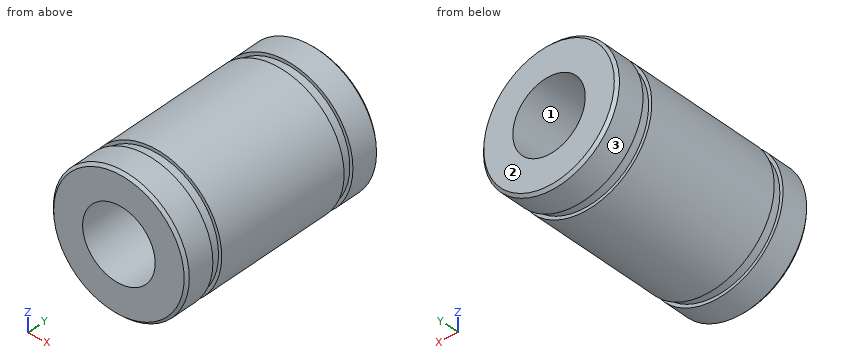
Autodesk Fusion 360 part; units mm, degrees
sketch "Sketch1" plane through (0, 0, 0) normal (0, 1, 0) x (1, 0, 0)
  circle A0 centre (0, 0) radius 4
  circle A1 centre (0, 0) radius 7.5
  circle A2 centre (0, 0) radius 7.15
  dimension "d1" = 8
  dimension "d2" = 15
  dimension "d6" = 0.35
extrude "Extrude1" add sketch "Sketch1" along normal blind 24 contours A1 | A2
extrude "Extrude2" cut sketch "Sketch1" along normal blind 1.1 from surface at 3.25 contours A1
extrude "Extrude3" cut sketch "Sketch1" against normal blind 1.1 from surface at 20.75 contours A1
chamfer "Chamfer1" distance 0.3 angle 45 2 edges at (-6.9925, 0, 2.7121) (-6.9925, 24, 2.7121)
Verification items for the finished model (mm, model axes). Face numbers are marked on the shaded views. Give positions to 0.01 mm unless a question says otherwise; leave off trailing zeros. Write each loop counter-clockwise with the first axis right and the second up, starting at its lowest first coordinate (ties: lowest second). Pieces come first, ordered by that corner, then holes. Notation, with made-up numbers: M -5.75,-13.5 L 9.25,-13.5 A21 ccw 9.25,23.5 Z; hole C 57.5,52 d3. An arc over 180 degrees is marked long. Write item = value, one per line.
(1) Sectioned sample at A-A (z = 0). Record the cut outline in (x, y), then the cut area to 3 significant figures.
Found:
outline = M -7.5,0.3 L -7.2,0 L -4,0 L -4,24 L -7.2,24 L -7.5,23.7 L -7.5,20.75 L -7.15,20.75 L -7.15,19.65 L -7.5,19.65 L -7.5,4.35 L -7.15,4.35 L -7.15,3.25 L -7.5,3.25 Z; M 4,0 L 7.2,0 L 7.5,0.3 L 7.5,3.25 L 7.15,3.25 L 7.15,4.35 L 7.5,4.35 L 7.5,19.65 L 7.15,19.65 L 7.15,20.75 L 7.5,20.75 L 7.5,23.7 L 7.2,24 L 4,24 Z
area = 166 mm2
(2) Sectioned sample at B-B (x = 0). Record the cut outline in (y, z), then the cut area to 3 significant figures.
Found:
outline = M 0,-7.2 L 0.3,-7.5 L 3.25,-7.5 L 3.25,-7.15 L 4.35,-7.15 L 4.35,-7.5 L 19.65,-7.5 L 19.65,-7.15 L 20.75,-7.15 L 20.75,-7.5 L 23.7,-7.5 L 24,-7.2 L 24,-4 L 0,-4 Z; M 0,4 L 24,4 L 24,7.2 L 23.7,7.5 L 20.75,7.5 L 20.75,7.15 L 19.65,7.15 L 19.65,7.5 L 4.35,7.5 L 4.35,7.15 L 3.25,7.15 L 3.25,7.5 L 0.3,7.5 L 0,7.2 Z
area = 166 mm2
(3) Material ranges on line 1 (X direction, y = 17, z = 0); line 2 (X direction, y = 13.75, z = 3.5), recorded low to high.
Found:
line_1 = -7.5 to -4, 4 to 7.5
line_2 = -6.63 to -1.94, 1.94 to 6.63
(4) Go/stop test with flat-tipped pins: pin 1 Ø5 at (x, y) = (3, 6) entering from -Z; pin 2 Ø1.5 at (x, z) = (-1, -3) entering from +Y; pin 3 Ø3 at (x, y) = (-3, 18) entering from +Z. Record where each tip stops, or that it passes through.
Found:
pin_1 = -7.48
pin_2 = through
pin_3 = 7.35
(5) Sectioned sample at C-C (y = 3.75). Record the cut outline in (x, z).
Found:
outline = C 0,0 d14.3; hole C 0,0 d8
(6) Draft check along X on the marked faces 1, 2 and 3. Enter one of: released by +X, released by -X, zero draft, split by the parting line, or undercut.
Found:
face_1 = undercut
face_2 = zero draft
face_3 = split by the parting line
(7) Sectioned sample at D-D (y = 18). Record the cut outline in (x, z), then the cut area to 3 significant figures.
Found:
outline = C 0,0 d15; hole C 0,0 d8
area = 126 mm2
